from build123d import *

# Parameters (mm, degrees)
F0_R     = 8
F1_DEPTH = 12.7
F2_R     = 4
F3_DEPTH = 5
F4_D     = 3.2639
F5_R     = 3.5


# Not quite as in the source:
# - a feature names something its author has since deleted; it is built from what else it names


with BuildPart() as f1:
    # F0 (on Top) → F1 (new body)
    with BuildSketch(Plane.XY):
        Circle(F0_R)
    extrude(amount=F1_DEPTH)

    # F2 (on face) → F3 (cut)
    with BuildSketch(Plane.XY.offset(12.7)):
        Circle(F2_R)
    extrude(amount=-F3_DEPTH, mode=Mode.SUBTRACT)

    # F4 (through all)
    with Locations(Plane(origin=(0, 0, 0), x_dir=(1, 0, 0), z_dir=(0, 0, -1))):
        with Locations((0, 0)):
            Hole(F4_D / 2)

    # F5
    f5_edges = [f1.edges().sort_by_distance(p)[0] for p in [
        (-8, 0, 12.7),
    ]]
    fillet(f5_edges, radius=F5_R)


solid = f1.part
Input: part model. Units: mm. Frame: model coordinates. A direction names the side the tool comes from. Coordinates: 2 decimals unless noted, no trailing zeros. Order: outer loops, then holes, each group sorted by start corner. A loop starts at its lowest first (then second) coordinate and runs counter-clockwise, first axis right, second up. Notation, with made-up numbers: M -33.75,-36.5 L -12.75,-36.5 A18 cw -12.75,-6.5 Z; hole C 27,13 d10. An arc over 180 degrees is marked long. Answer in a Markdown table with one row per item.
(1) Access query for faces 1 (the flat face through (2, 0, 0)), 2 (the flat face through (2, 0, 7.7)). Directions: +Z, -Z, +X, -X, +Y, -Y. A direction counts if a zero-diameter tool reaches every point of the face in a straight line with its end or side. Return the directions, or none.
Numbers:
| item | result |
|---|---|
| face 1 | -Z, +X, -X, +Y, -Y |
| face 2 | +Z |
(2) Section query A-A, the plane x = 0. Output: boundary loops of the cut face in (y, z), plus the area to 3 significant figures.
Numbers:
| item | result |
|---|---|
| outline | M -8,0 L -1.63,0 L -1.63,7.7 L -4,7.7 L -4,12.7 L -4.5,12.7 A3.5 ccw -8,9.2 Z; M 1.63,0 L 8,0 L 8,9.2 A3.5 ccw 4.5,12.7 L 4,12.7 L 4,7.7 L 1.63,7.7 Z |
| area | 133 mm^2 |
(3) Material intervals for line 1 (Y direction, x = 0, z = 9.1); line 2 (Y direction, x = 0, z = 6); line 3 (X direction, y = 1.5, z = 11), sorted ascending. Write a range as [from, to].
Numbers:
| item | result |
|---|---|
| line 1 | y = [-8, -4], [4, 8] |
| line 2 | y = [-8, -1.63], [1.63, 8] |
| line 3 | x = [-7.35, -3.71], [3.71, 7.35] |
(4) Section query D-D, the plane z = 11.25. Output: boundary loops of the cut face in (x, y).
Numbers:
| item | result |
|---|---|
| outline | C 0,0 d14.67; hole C 0,0 d8 |
(5) Draft query along Y for faces 3 (the flat face through (-3, -3, 12.7)), 4 (the cylindrical face through (0.354, 1.593, 3.904)), 5 (the cylindrical face through (-1.73, -7.81, 4.54)). Return one class per face: pulls with the +Y half, pulls with the -Y half, needs draft (parallel to the pull), parting line crosses it, or undercut.
Numbers:
| item | result |
|---|---|
| face 3 | needs draft |
| face 4 | undercut |
| face 5 | parting line crosses it |
(6) Section query C-C, the plane z = 7. Output: boundary loops of the cut face in (x, y), plus the area to 3 significant figures.
Numbers:
| item | result |
|---|---|
| outline | C 0,0 d16; hole C 0,0 d3.26 |
| area | 193 mm^2 |
(7) Contact query for flat-ended pins moving along their axis: pin 1 Ø6.5 at (x, y) = (0, 0) entering from +Z; pin 2 Ø2 at (y, z) = (1.5, 2.5) entering from -X; pin 3 Ø4 at (y, z) = (4, 10.5) entering from -X; pin 4 Ø2.5 at (x, y) = (0, 0) entering from -Z. Output: stop coordinate, or through.
Numbers:
| item | result |
|---|---|
| pin 1 | stops at z = 7.7 |
| pin 2 | stops at x = -7.98 |
| pin 3 | stops at x = -7.66 |
| pin 4 | passes through |
